from build123d import *

# Parameters (mm, degrees)
PAD_DEPTH       = 40
POCKET_DEPTH    = 32
POCKET001_DEPTH = 1
SKETCH007_R     = 4
SKETCH007_R_2   = 1.95
SKETCH007_R_3   = 2
PAD005_DEPTH    = 5.5
SKETCH008_W     = 16
SKETCH008_H     = 8
POCKET002_DEPTH = 39
SKETCH013_R     = 1.95
POCKET003_DEPTH = 8
SKETCH018_W     = 40.6
SKETCH018_H     = 12
SKETCH018_H_2   = 9
PAD012_DEPTH    = 16.5
SKETCH019_W     = 35.9
SKETCH019_H     = 56.1
POCKET006_DEPTH = 11.9


with BuildPart() as part:
    # Sketch → Pad (new body, symmetric)
    with BuildSketch(Plane.XZ):
        Polygon((-59, 16.5), (-59, -5.7), (-41, -5.7), (-41, 0), (59, 0), (59, 16.5), align=None)
    extrude(amount=PAD_DEPTH, both=True)

    # Sketch001 → Pocket (cut, symmetric)
    with BuildSketch(Plane.XZ):
        Polygon((-42, 1), (51, 1), (51, 17.5), (-58, 17.5), (-58, -4.7), (-42, -4.7), align=None)
    extrude(amount=POCKET_DEPTH, both=True, mode=Mode.SUBTRACT)

    # Sketch004 → Pocket001 (cut)
    with BuildSketch(Plane.XY):
        with BuildLine():
            ThreePointArc((-3.5, 5), (-8.5, 0), (-3.5, -5))
            Line((-3.5, -5), (21.5, -5))
            ThreePointArc((21.5, -5), (26.5, 0), (21.5, 5))
            Line((21.5, 5), (-3.5, 5))
        make_face()
    extrude(amount=POCKET001_DEPTH, mode=Mode.SUBTRACT)

    # Sketch007 → Pad005 (join)
    with BuildSketch(Plane.XY):
        with Locations((13.6, 17)):
            Circle(SKETCH007_R)
        with Locations((13.6, 17)):
            Circle(SKETCH007_R_2, mode=Mode.SUBTRACT)
        with Locations((35.6, 17)):
            Circle(SKETCH007_R)
        with Locations((35.6, 17)):
            Circle(SKETCH007_R_2, mode=Mode.SUBTRACT)
        with Locations((24.6, -14)):
            Circle(SKETCH007_R_3)
    extrude(amount=PAD005_DEPTH)

    # Sketch008 → Pocket002 (cut, symmetric)
    with BuildSketch(Plane.XZ):
        with Locations((-50, -0.7)):
            Rectangle(SKETCH008_W, SKETCH008_H)
    extrude(amount=POCKET002_DEPTH, both=True, mode=Mode.SUBTRACT)

    # Sketch013 (on DatumPlane) → Pocket003 (cut)
    with BuildSketch(Plane.XY.offset(16.5)):
        with Locations((-55, 36)):
            Circle(SKETCH013_R)
        with Locations((1, 36)):
            Circle(SKETCH013_R)
        with Locations((55, 36)):
            Circle(SKETCH013_R)
        with Locations((55, -36)):
            Circle(SKETCH013_R)
        with Locations((1, -36)):
            Circle(SKETCH013_R)
        with Locations((-55, -36)):
            Circle(SKETCH013_R)
    extrude(amount=-POCKET003_DEPTH, mode=Mode.SUBTRACT)

    # Sketch018 → Pad012 (join)
    with BuildSketch(Plane.XY):
        with Locations((-21.7, 20.8)):
            Rectangle(SKETCH018_W, SKETCH018_H)
        with Locations((-21.7, -27.5)):
            Rectangle(SKETCH018_W, SKETCH018_H_2)
    extrude(amount=PAD012_DEPTH)

    # Sketch019 (on DatumPlane) → Pocket006 (cut)
    with BuildSketch(Plane.XY.offset(16.5)):
        with Locations((-21.55, -3.95)):
            Rectangle(SKETCH019_W, SKETCH019_H)
    extrude(amount=-POCKET006_DEPTH, mode=Mode.SUBTRACT)


solid = part.part
For this review, take the finished solid that the model builds, in its own axes (mm). A direction names the side the tool comes from. Round coordinates to 2 decimals unless told otherwise and drop trailing zeros. Order: outer loops, then holes, each group sorted by start corner. A loop starts at its lowest first (then second) coordinate and runs counter-clockwise, first axis right, second up. Notation, with made-up numbers: (89, -33) -> (117, -33) arc R21 ccw to (117, -6) -> close; hole circle Ø6 at (22, 64.25). An arc over 180 degrees is marked (long way). Write item = value, one per line. Start each with the question number.
1) Take a section at B-B on x = 20. State the section outline as (y, z) points, plus the area to 3 significant figures.
2) The part is to be moulded in two halves that separate along X. For faces 4 (the face through (-55, 36, 8.5)), 5 (the face through (-23, 25, 16.5)), 6 (the face through (59, -1, 8)), say which applies: +X half, -X half, draft (parallel to the pull), parting line (faces both ways), or undercut.
3) Take a section at C-C on y = 36. State the section outline as (x, z) points.
4) Insertion check: pin 1 (8 mm diameter, centred on x = 0, y = -4.5, fed in from -Z); pin 2 (1.2 mm diameter, centred on x = 1, y = 36.5, fed in from +Z); pin 3 (6.5 mm diameter, centred on x = 15, y = 17.5, fed in from +Z). Each pin has a flat end and moves straight along its axis. Give the tip position at first contact, or say it passes through.
5) Take a section at A-A on z = 13. Count the separate pieces of the cut face and the enclosed holes in it, plus the area to 3 significant figures.
6) To check wall thickness, follow line 1 (Y direction, x = -55, z = 13.25); line 2 (X direction, y = -26, z = 10); line 3 (Y direction, x = -33, z = 15.75). State the ranges of each line that lie inside material, in increasing order. Write a range as from..to.
7) Take a section at D-D on z = -1.25. State the section outline as (x, y) points.
8) Tool access review of faces 1 (the face through (24, -32, 9)), 2 (the face through (-41, -1, -3)), 3 (the face through (-1, 40, 8)): name each direction out of +Z, -Z, +X, -X, +Y, -Y from which nothing blocks a thin tool from reaching the whole face with its end or side.
Verdict:
q1.outline = (-40, 0) -> (-5, 0) -> (-5, 1) -> (-32, 1) -> (-32, 16.5) -> (-40, 16.5) -> close; (5, 0) -> (40, 0) -> (40, 16.5) -> (32, 16.5) -> (32, 1) -> (5, 1) -> close
q1.area = 318 mm2
q2.face_4 = undercut
q2.face_5 = draft
q2.face_6 = +X half
q3.outline = (-59, -5.7) -> (-41, -5.7) -> (-41, 0) -> (59, 0) -> (59, 16.5) -> (56.95, 16.5) -> (56.95, 8.5) -> (53.05, 8.5) -> (53.05, 16.5) -> (2.95, 16.5) -> (2.95, 8.5) -> (-0.95, 8.5) -> (-0.95, 16.5) -> (-53.05, 16.5) -> (-53.05, 8.5) -> (-56.95, 8.5) -> (-56.95, 16.5) -> (-59, 16.5) -> close; hole (-58, -4.7) -> (-42, -4.7) -> (-42, 3.3) -> (-58, 3.3) -> close
q4.pin_1 = 0
q4.pin_2 = 8.5
q4.pin_3 = 5.5
q5.separate_pieces = 2
q5.enclosed_holes = 7
q5.area = 2,590 mm2
q6.line_1 = -40..-37.95, -34.05..-32, 32..34.05, 37.95..40
q6.line_2 = -59..-58, -42..-39.5, -3.6..-1.4, 51..59
q6.line_3 = -40..-32, 24.1..26.8, 32..40
q7.outline = (-59, -40) -> (-41, -40) -> (-41, 40) -> (-59, 40) -> close; hole (-58, -39) -> (-42, -39) -> (-42, 39) -> (-58, 39) -> close
q8.face_1 = +Z
q8.face_2 = -Z, +X, +Y, -Y
q8.face_3 = +Z, -Z, +X, -X, +Y
